from build123d import *

# Parameters (mm, degrees)
SKETCH1_W           = 40
SKETCH1_H           = 12
SKETCH1_R           = 2
BOSS_EXTRUDE1_DEPTH = 14
SKETCH2_R           = 3.5
CUT_EXTRUDE1_DEPTH  = 5


with BuildPart() as part:
    # Sketch1 → Boss-Extrude1 (new body)
    with BuildSketch(Plane.XY):
        with Locations((27.119550003, 16.407464025)):
            Rectangle(SKETCH1_W, SKETCH1_H)
        with Locations((13.119550003, 16.407464025)):
            Circle(SKETCH1_R, mode=Mode.SUBTRACT)
        with Locations((41.119550003, 16.407464025)):
            Circle(SKETCH1_R, mode=Mode.SUBTRACT)
    extrude(amount=BOSS_EXTRUDE1_DEPTH)

    # Sketch2 → Cut-Extrude1 (cut)
    with BuildSketch(Plane.XY):
        with Locations((13.119550003, 16.407464025)):
            Circle(SKETCH2_R)
        with Locations((41.119550003, 16.407464025)):
            Circle(SKETCH2_R)
    extrude(amount=CUT_EXTRUDE1_DEPTH, mode=Mode.SUBTRACT)

    # Sketch3 → Cut-Revolve1 (revolve, cut)
    with BuildSketch(Plane.XY.offset(14)):
        Polygon((35.119550003, 22.407464025), (35.119550003, 18.407464025), (33.119550003, 18.407464025), (33.119550003, 12.407464025), (35.119550003, 12.407464025), (35.119550003, 10.407464025), (27.119550003, 10.407464025), (27.119550003, 22.407464025), align=None)
    revolve(axis=Axis((27.119550003, 22.407464025, 14), (0, -1, 0)), mode=Mode.SUBTRACT)


solid = part.part
Input: part model. Units: mm. Frame: model coordinates. A direction names the side the tool comes from. Round coordinates to 2 decimals unless told otherwise and drop trailing zeros. Order: outer loops, then holes, each group sorted by start corner. A loop starts at its lowest first (then second) coordinate and runs counter-clockwise, first axis right, second up.
1. Pin query (flat end, axial travel): P1, Ø1, axis at x = 24, z = 11, coming from the -Y side; P2, Ø5.5, axis at x = 13.5, y = 16, coming from the -Z side. Return the tip coordinate at first contact, or that it passes through.
The answers:
P1: passes through
P2: stops at z = 5
2. Mould query, pull axis Y, two halves, no side actions, for faces 5 (the face through (47.12, 16, 7)), 6 (the face through (28.3, 12.407, 7.9)), 7 (the face through (15, 19.36, 2.46)), 8 (the face through (25.9, 18.407, 7.9)). Classes: released by +Y, released by -Y, zero draft, split by the parting line, or undercut.
The answers:
face 5: zero draft
face 6: released by -Y
face 7: undercut
face 8: released by +Y
3. Set-up query: faces 1 (the face through (27, 20, 6)), 2 (the face through (27, 11, 6)), 3 (the face through (43, 15, 5)), 4 (the face through (27, 15, 8)). Return all of +Z, -Z, +X, -X, +Y, -Y with unobstructed straight access to the full face (end or side cutting, diameter ignored); none if empty.
The answers:
face 1: +Z, +Y
face 2: +Z, -Y
face 3: -Z
face 4: +Z, +Y, -Y
4. Cut plane C-C, the plane y = 17.25. Output: boundary loops of the cut face in (x, z).
The answers:
outline: (7.12, 0) - (9.72, 0) - (9.72, 5) - (11.31, 5) - (11.31, 14) - (7.12, 14) - close; (14.93, 5) - (16.52, 5) - (16.52, 0) - (37.72, 0) - (37.72, 5) - (39.31, 5) - (39.31, 14) - (33.12, 14) arc R6 cw to (21.12, 14) - (14.93, 14) - close; (42.93, 5) - (44.52, 5) - (44.52, 0) - (47.12, 0) - (47.12, 14) - (42.93, 14) - close
5. Cut plane D-D, the plane y = 12. Output: boundary loops of the cut face in (x, z), then the cut area to 3 significant figures.
The answers:
outline: (7.12, 0) - (47.12, 0) - (47.12, 14) - (35.12, 14) arc R8 cw to (19.12, 14) - (7.12, 14) - close
area: 459 mm2
6. Cut plane B-B, the plane x = 42. Output: boundary loops of the cut face in (y, z), then the cut area to 3 significant figures.
The answers:
outline: (10.41, 0) - (13.02, 0) - (13.02, 5) - (14.61, 5) - (14.61, 14) - (10.41, 14) - close; (18.2, 5) - (19.79, 5) - (19.79, 0) - (22.41, 0) - (22.41, 14) - (18.2, 14) - close
area: 102 mm2
7. Material intervals for line 1 (X direction, y = 16.25, z = 4); line 2 (Y direction, x = 41, z = 8); line 3 (X direction, y = 18.75, z = 2.5), sorted ascending.
The answers:
line 1: x = 7.12 to 9.62, 16.62 to 37.62, 44.62 to 47.12
line 2: y = 10.41 to 14.41, 18.4 to 22.41
line 3: x = 7.12 to 10.52, 15.72 to 38.52, 43.72 to 47.12
8. Cut plane A-A, the plane z = 12. Output: boundary loops of the cut face in (x, y).
The answers:
outline: (7.12, 10.41) - (19.37, 10.41) - (19.37, 12.41) - (21.46, 12.41) - (21.46, 18.41) - (19.37, 18.41) - (19.37, 22.41) - (7.12, 22.41) - close; (32.78, 12.41) - (34.87, 12.41) - (34.87, 10.41) - (47.12, 10.41) - (47.12, 22.41) - (34.87, 22.41) - (34.87, 18.41) - (32.78, 18.41) - close; hole circle Ø4 at (13.12, 16.41); hole circle Ø4 at (41.12, 16.41)
